Geometry check sheet. Reference: the model listing, model coordinates, mm. A direction names the side the tool comes from. Coordinates: 2 decimals unless noted, no trailing zeros. Write each loop counter-clockwise with the first axis right and the second up, starting at its lowest first coordinate (ties: lowest second). Pieces come first, ordered by that corner, then holes. Notation, with made-up numbers: (-29.75, 63) -> (29.25, 63) arc R13 cw to (29.25, 77) -> close; hole circle Ø11 at (-9.5, 37.25). An arc over 180 degrees is marked (long way). Answer in a Markdown table with one row per item. Add a question column.
Q1. Gauge pin test, flat ends, axial feed: P1, Ø3, axis at y = 7.5, z = 15.5, coming from the +X side; P2, Ø4, axis at y = 6, z = 20, coming from the +X side; P3, Ø8, axis at y = 2.5, z = -1, coming from the -X side; P4, Ø1, axis at x = 3, y = -2, coming from the +Z side. Record the tip position at first contact, or that the pin passes through.
Q2. Tool access check on faces 1 (the face through (-25.983, -2.465, 9.268)), 2 (the face through (-18, 0, 6)). Record the directions out of +Z, -Z, +X, -X, +Y, -Y that give a thin tool (end or side, any length) a straight path to the whole face; none if there is none.
Q3. Section check B-B, the plane z = 14. Record the boundary of the cut face in (x, y), and give its area (3 significant figures).
Q4. Thickness scan on line 1 (Z direction, x = -10.5, y = 7.25); line 2 (Y direction, x = -2.5, z = 20); line 3 (Z direction, x = -8, y = 4). Record the ranges inside material, lowest first.
Q5. Release check for a two-part mould opening along Z. For faces 3 (the face through (-18, -5, 10)), 4 (the face through (2.8, -2.5, 8.4)), 5 (the face through (-14.613, 4.93, 3.277)), 6 (the face through (-5.944, 2.395, 5.883)) record: pulls with the +Z half, pulls with the -Z half, needs draft (parallel to the pull), parting line crosses it, or undercut.
Q6. Section check C-C, the plane z = 10.5. Record the boundary of the cut face in (x, y).
Q7. Section check D-D, the plane y = 4. Record the boundary of the cut face in (x, z), and give its area (3 significant figures).
Q8. Section check A-A, the plane x = -10. Record the boundary of the cut face in (y, z).
Autodesk Inventor part; units mm, degrees
ref_plane "YZ Plane" through (0, 0, 0) normal (1, 0, 0) x (0, 1, 0)
ref_plane "XZ Plane" through (0, 0, 0) normal (0, 1, 0) x (-1, 0, 0)
ref_plane "XY Plane" through (0, 0, 0) normal (0, 0, 1) x (1, 0, 0)
sketch "Boceto1" plane through (0, 0, 0) normal (0, 1, 0) x (-1, 0, 0)
  circle A0 centre (10.3662, 9.9379) radius 6
  circle A1 centre (10.3662, 9.9379) radius 7.9
  circle A2 centre (10.3662, 9.9379) radius 17
  line L0 (18.2662, 9.9379) -> (22.6162, 9.9379)
  line L1 (2.4662, 9.9379) -> (-1.8838, 9.9379)
  line L2 (22.6162, 9.9379) -> (24.3662, 9.9379)
  line L3 (-1.8838, 9.9379) -> (-3.6338, 9.9379)
  circle A3 centre (24.3662, 9.9379) radius 1.75
  circle A4 centre (-3.6338, 9.9379) radius 1.75
  dimension "d0" = 12
  dimension "d1" = 15.8
  dimension "d35" = 34
  dimension "d40" = 14
  dimension "d41" = 14
extrude "Extrusión6" add sketch "Boceto1" along normal blind 10 contours A1
extrude "Extrusión8" add sketch "Boceto1" against normal blind 5 contours A1 | A2
thread "Thread3"
properties part number "Tuerca de mesa" material "Brass, Soft Yellow"
Calculated:
| question | item | result |
|---|---|---|
| 1 | P1 | stops at x = -3.59 |
| 1 | P2 | passes through |
| 1 | P3 | stops at x = -25.46 |
| 1 | P4 | stops at z = 21.05 |
| 2 | face 1 | +Y, -Y |
| 2 | face 2 | +Y |
| 3 | outline | (-26.87, -5) -> (-14.78, -5) -> (-14.78, 10) -> (-17.14, 10) -> (-17.14, 0) -> (-26.87, 0) -> close; (-5.95, -5) -> (6.14, -5) -> (6.14, 0) -> (-3.59, 0) -> (-3.59, 10) -> (-5.95, 10) -> close |
| 3 | area | 168 mm² |
| 4 | line 1 | z = 2.04 to 3.94, 15.94 to 17.84 |
| 4 | line 2 | y = -5 to 0 |
| 4 | line 3 | z = 2.4 to 4.42, 15.45 to 17.48 |
| 5 | face 3 | needs draft |
| 5 | face 4 | undercut |
| 5 | face 5 | parting line crosses it |
| 5 | face 6 | undercut |
| 6 | outline | (-27.36, -5) -> (-26.02, -5) -> (-26.02, 0) -> (-27.36, 0) -> close; (-22.71, -5) -> (-16.34, -5) -> (-16.34, 10) -> (-18.25, 10) -> (-18.25, 0) -> (-22.71, 0) -> close; (-4.39, -5) -> (1.98, -5) -> (1.98, 0) -> (-2.49, 0) -> (-2.49, 10) -> (-4.39, 10) -> close; (5.29, -5) -> (6.62, -5) -> (6.62, 0) -> (5.29, 0) -> close |
| 7 | outline | circle Ø15.8 at (-10.37, 9.94); hole circle Ø12 at (-10.37, 9.94) |
| 7 | area | 83.0 mm² |
| 8 | outline | (-5, -7.06) -> (0, -7.06) -> (0, 2.05) -> (10, 2.05) -> (10, 3.95) -> (-5, 3.95) -> close; (-5, 15.93) -> (10, 15.93) -> (10, 17.83) -> (0, 17.83) -> (0, 26.93) -> (-5, 26.93) -> close |
